Design review of the part shown in the three views and the two pictorial views. Dimensions are in mm from the part's minimum x, y and z. A direction names the side the tool comes from. Give positions to 0.01 mm unless a question says otherwise; leave off trailing zeros. Order: outer loops, then holes, each group sorted by start corner. A loop starts at its lowest first (then second) coordinate and runs counter-clockwise, first axis right, second up.
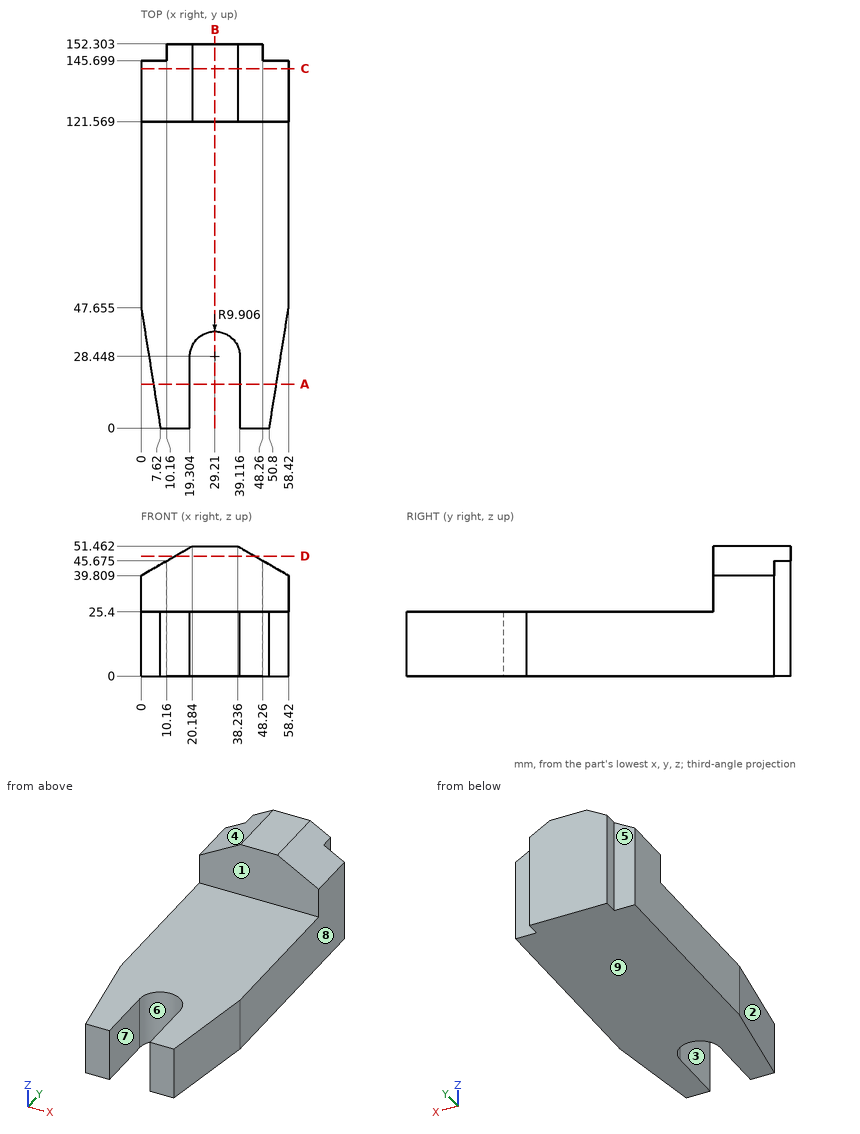
Item 1: For the marked faces 1, 2, 3, 4 and 5, list the 3-axis set-ups (+Z, -Z, +X, -X, +Y, -Y) from which the entire face can be reached by the end or side of a thin tool; tool diameter is ignored.
Values found:
face 1: +Z, +X, -X, -Y
face 2: +Z, -Z, -X, -Y
face 3: +Z, -Z, -Y
face 4: +Z, -X, +Y, -Y
face 5: +Z, -Z, -X, +Y
Item 2: Take a section at B-B (x = 29.21). Give the boundary of the cut face in (y, z), and give its area (3 significant figures).
Values found:
outline: (38.35, 0) - (152.3, 0) - (152.3, 51.46) - (121.57, 51.46) - (121.57, 25.4) - (38.35, 25.4) - close
area: 3,700 mm2
Item 3: Take a section at A-A (y = 17.5). Give the boundary of the cut face in (x, z), and give its area (3 significant figures).
Values found:
outline: (4.82, 0) - (19.3, 0) - (19.3, 25.4) - (4.82, 25.4) - close; (39.12, 0) - (53.6, 0) - (53.6, 25.4) - (39.12, 25.4) - close
area: 736 mm2
Item 4: Take a section at D-D (z = 47.5). Give the boundary of the cut face in (x, y).
Values found:
outline: (13.32, 121.57) - (45.1, 121.57) - (45.1, 152.3) - (13.32, 152.3) - close
Item 5: Draft analysis for pull direction X (two halves, no side actions). For the marked faces 6, 7, 8 and 9, state which applies: released by +X, released by -X, zero draft, split by the parting line, or undercut.
Values found:
face 6: undercut
face 7: undercut
face 8: released by +X
face 9: zero draft
Item 6: For line 1 (X direction, y = 146.5, z = 45); line 2 (Z direction, x = 13, y = 100); line 3 (Y direction, x = 8, z = 18), list the stretches that pass through material, from the lowest coordinate up.
Values found:
line 1: x = 10.16 to 48.26
line 2: z = 0 to 25.4
line 3: y = 0 to 145.7
Item 7: Clearance check with flat-ended pins moving along their axes: pin 1 Ø7.5 at (y, z) = (149.5, 29) entering from -X; pin 2 Ø3 at (x, z) = (53.5, 21.5) entering from +Y; pin 3 Ø12.5 at (y, z) = (16.5, 7.5) entering from +X. State where each tip first meets the part, or that it passes through.
Values found:
pin 1: stops at x = 10.16
pin 2: stops at y = 145.7
pin 3: stops at x = 54.44
Item 8: Take a section at C-C (y = 142.5). Give the boundary of the cut face in (x, z).
Values found:
outline: (0, 0) - (58.42, 0) - (58.42, 39.81) - (38.24, 51.46) - (20.18, 51.46) - (0, 39.81) - close
